from build123d import *

# Parameters (mm, degrees)
SKETCH1_W               = 100
SKETCH1_H               = 76
BOSS_EXTRUDE1_DEPTH     = 3
CUT_EXTRUDE1_START      = -4
SKETCH2_W               = 14
SKETCH2_H               = 14
CUT_EXTRUDE1_DEPTH      = 5
LPATTERN1_COUNT         = 4
LPATTERN1_PITCH         = 19.05
LPATTERN1_COUNT_DIR2    = 4
LPATTERN1_PITCH_DIR2    = 19.05
SKETCH4_R               = 2
CUT_EXTRUDE2_DEPTH      = 1
CUT_EXTRUDE2_DEPTH_BACK = 4


with BuildPart() as part:
    # Sketch1 → Boss-Extrude1 (new body)
    with BuildSketch(Plane(origin=(0, 0, 0), x_dir=(1, 0, 0), z_dir=(0, 1, 0))):
        with Locations((50, 38)):
            Rectangle(SKETCH1_W, SKETCH1_H)
    extrude(amount=BOSS_EXTRUDE1_DEPTH)

    # Sketch2 → Cut-Extrude1 (cut)
    with BuildSketch(Plane(origin=(0, 3, 0), x_dir=(1, 0, 0), z_dir=(0, 1, 0)).offset(CUT_EXTRUDE1_START)):
        with Locations((9.5, 9.5)):
            Rectangle(SKETCH2_W, SKETCH2_H)
    cut_extrude1 = extrude(amount=CUT_EXTRUDE1_DEPTH, mode=Mode.SUBTRACT)

    # LPattern1: Cut-Extrude1 4 × 4
    with Locations(*[(j * LPATTERN1_PITCH_DIR2, 0, -i * LPATTERN1_PITCH) for i in range(LPATTERN1_COUNT) for j in range(LPATTERN1_COUNT_DIR2) if (i, j) != (0, 0)]):
        add(cut_extrude1, mode=Mode.SUBTRACT)

    # Sketch4 → Cut-Extrude2 (cut, two sides)
    with BuildSketch(Plane(origin=(0, 3, 0), x_dir=(1, 0, 0), z_dir=(0, 1, 0))) as cut_extrude2_sk:
        with Locations((19.025, 57.125)):
            Circle(SKETCH4_R)
        with Locations((57.317897374, 57.125)):
            Circle(SKETCH4_R)
        with Locations((19.025, 19.025)):
            Circle(SKETCH4_R)
        with Locations((57.317897374, 19.025)):
            Circle(SKETCH4_R)
    extrude(amount=CUT_EXTRUDE2_DEPTH, mode=Mode.SUBTRACT)
    extrude(cut_extrude2_sk.sketch, amount=-CUT_EXTRUDE2_DEPTH_BACK, mode=Mode.SUBTRACT)


solid = part.part
Geometry check sheet. Reference: the model listing, model coordinates, mm. Round coordinates to 2 decimals unless told otherwise and drop trailing zeros. Loops run counter-clockwise (first coordinate to the right, second up) from the corner with the lowest first, then second, coordinate; pieces in that order, holes last.
Item 1: Cross-section at D-D on y = 1.75. Count the separate pieces of the cut face and the enclosed holes in it, then the cut area to 3 significant figures.
Item 2: Mould release check, pull along X, two halves, no side actions. Record for faces 1 (the flat face through (60, 3, -39)), 2 (the flat face through (67, 1, -59.65)): pulls with the +X half, pulls with the -X half, needs draft (parallel to the pull), parting line crosses it, or undercut.
Item 3: Cross-section at B-B on x = 8. Record the boundary of the cut face in (y, z).
Item 4: Cross-section at A-A on z = -42. Record the boundary of the cut face in (x, y).
Item 5: Gauge pin test, flat end, axial feed: pin 1 (2 mm diameter, centred on x = 44.5, z = -43, fed in from -Y). Record the tip position at first contact, or that the pin passes through.
Item 6: Cross-section at C-C on x = 58. Record the boundary of the cut face in (y, z).
Item 7: Thickness scan on line 1 (X direction, y = 0.55, z = -71.5); line 2 (Z direction, x = 66, y = 0.7); line 3 (Z direction, x = 18, y = 2.55). Record the ranges inside material, lowest first.
Answer sheet:
1. separate pieces: 1
1. enclosed holes: 20
1. area: 4,410 mm2
2. face 1: needs draft
2. face 2: undercut
3. outline: (0, -76) - (3, -76) - (3, -73.65) - (0, -73.65) - close; (0, -59.65) - (3, -59.65) - (3, -54.6) - (0, -54.6) - close; (0, -40.6) - (3, -40.6) - (3, -35.55) - (0, -35.55) - close; (0, -21.55) - (3, -21.55) - (3, -16.5) - (0, -16.5) - close; (0, -2.5) - (3, -2.5) - (3, 0) - (0, 0) - close
4. outline: (0, 0) - (2.5, 0) - (2.5, 3) - (0, 3) - close; (16.5, 0) - (21.55, 0) - (21.55, 3) - (16.5, 3) - close; (35.55, 0) - (40.6, 0) - (40.6, 3) - (35.55, 3) - close; (54.6, 0) - (59.65, 0) - (59.65, 3) - (54.6, 3) - close; (73.65, 0) - (100, 0) - (100, 3) - (73.65, 3) - close
5. pin 1: passes through
6. outline: (0, -76) - (3, -76) - (3, -59.01) - (0, -59.01) - close; (0, -55.24) - (3, -55.24) - (3, -20.91) - (0, -20.91) - close; (0, -17.14) - (3, -17.14) - (3, 0) - (0, 0) - close
7. line 1: x = 0 to 2.5, 16.5 to 21.55, 35.55 to 40.6, 54.6 to 59.65, 73.65 to 100
7. line 2: z = -76 to -73.65, -59.65 to -54.6, -40.6 to -35.55, -21.55 to -16.5, -2.5 to 0
7. line 3: z = -76 to -58.84, -55.41 to -20.74, -17.31 to 0
